Work out the finished part from the listing and answer in its coordinate system (mm). A direction names the side the tool comes from. Coordinates: 2 decimals unless noted, no trailing zeros. Loops run counter-clockwise (first coordinate to the right, second up) from the corner with the lowest first, then second, coordinate; pieces in that order, holes last.
```python
from build123d import *

# Parameters (mm, degrees)
SKETCH1_R           = 3
SKETCH1_R_2         = 8
SKETCH1_R_3         = 1.8
BOSS_EXTRUDE1_DEPTH = 6.2


with BuildPart() as part:
    # Sketch1 → Boss-Extrude1 (new body)
    with BuildSketch(Plane.XY):
        with BuildLine():
            Line((41.889296616, 14.900574245), (50.746753734, 13.965723579))
            ThreePointArc((50.746753734, 13.965723579), (58.138171033, 17.219277376), (59.076989694, 25.240329771))
            ThreePointArc((59.076989694, 25.240329771), (47.870351378, 40.981444556), (31.114327774, 50.604703359))
            ThreePointArc((31.114327774, 50.604703359), (-11.412690469, 54.769217303), (-51.987221097, 41.367802402))
            ThreePointArc((-51.987221097, 41.367802402), (-62.079231834, 16.80974691), (-41, 0.666241851))
            Line((-41, 0.666241851), (-35, 0.666241851))
            ThreePointArc((-35, 0.666241851), (-26.181808949, -1.950576316), (-20.218406631, -8.953865794))
            ThreePointArc((-20.218406631, -8.953865794), (3.76322615, -21.789763842), (22.050412422, -1.653780932))
            ThreePointArc((22.050412422, -1.653780932), (28.467658292, 10.820459281), (41.889296616, 14.900574245))
        make_face()
        with Locations(Location((-41, 22.5, 0), (0, 0, 180))):
            Circle(SKETCH1_R, mode=Mode.SUBTRACT)
        with Locations(Location((6, 41.25, 0), (0, 0, 180))):
            Circle(SKETCH1_R, mode=Mode.SUBTRACT)
        with Locations(Location((51.6, 22.050001086, 0), (0, 0, 180))):
            Circle(SKETCH1_R, mode=Mode.SUBTRACT)
        with Locations(Location((0, 0, 0), (0, 0, 180))):
            Circle(SKETCH1_R_2, mode=Mode.SUBTRACT)
        with Locations(Location((25.2, 42.25, 0), (0, 0, 180))):
            Circle(SKETCH1_R_3, mode=Mode.SUBTRACT)
        with Locations(Location((-32.4, 15.5, 0), (0, 0, 180))):
            Circle(SKETCH1_R_3, mode=Mode.SUBTRACT)
        with Locations(Location((42, 20.450001086, 0), (0, 0, 180))):
            Circle(SKETCH1_R_3, mode=Mode.SUBTRACT)
        with Locations(Location((-41, 33.5, 0), (0, 0, 180))):
            Circle(SKETCH1_R_3, mode=Mode.SUBTRACT)
    extrude(amount=BOSS_EXTRUDE1_DEPTH)


solid = part.part
```
1. A cutting plane is placed at B-B, the plane y = 3. Give the vertices of the cut face in (x, z).
2. Straight lines are drawn through the part: probe 1 along Y at (x, z) = (-41, 1.75); probe 2 along Y at (x, z) = (6, 3); probe 3 along X at (y, z) = (24, 2.75). For each, find the intervals that lie inside material, in ascending order.
3. A cutting plane is placed at D-D, the plane y = 27.5. Give the vertices of the cut face in (x, z), then the cut area to 3 significant figures.
4. A cutting plane is placed at A-A, the plane z = 5.25. Count the separate pieces of the cut face and the enclosed holes in it, then the cut area to 3 significant figures.
5. For faces 4 (the flat face through (-2, 26, 0)), 5 (the flat face through (-38, 0.666, 3)), determine the directions among +Z, -Z, +X, -X, +Y, -Y from which every point of the face is accessible in a straight line to the end or side of a thin tool.
6. A cutting plane is placed at C-C, the plane x = -3. Give the vertices of the cut face in (y, z), then the cut area to 3 significant figures.
7. Determine the mould class of faces 1 (the cylindrical face through (40.283, 19.909, 3.057)), 2 (the flat face through (46.26, 14.44, 3.06)), 3 (the flat face through (-2, 26, 6.2)) for opening direction Y: released by +Y, released by -Y, zero draft, split by the parting line, or undercut.
8. Each of these flat-tipped pins is pushed along its axis until it touches: P1, Ø4, axis at x = 42, y = 20.45, coming from the +Z side; P2, Ø3, axis at x = -37, z = 4, coming from the -Y side; P3, Ø5, axis at x = 51.6, y = 22.05, coming from the +Z side; P4, Ø3, axis at y = 32, z = 4.5, coming from the -X side. Where does it stop, or does it pass through?
Answers below:
1. outline: (-50.82, 0) - (-7.42, 0) - (-7.42, 6.2) - (-50.82, 6.2) - close; (7.42, 0) - (23.03, 0) - (23.03, 6.2) - (7.42, 6.2) - close
2. probe 1: y = 0.67 to 19.5, 25.5 to 31.7, 35.3 to 46.92
2. probe 2: y = -21.28 to -5.29, 5.29 to 38.25, 44.25 to 55.23
2. probe 3: x = -62.78 to -43.6, -38.4 to 49.32, 53.88 to 59.49
3. outline: (-62.25, 0) - (58.04, 0) - (58.04, 6.2) - (-62.25, 6.2) - close
3. area: 746 mm2
4. separate pieces: 1
4. enclosed holes: 8
4. area: 5,730 mm2
5. face 4: -Z, +X, -X, +Y, -Y
5. face 5: +Z, -Z, -X, -Y
6. outline: (-21.91, 0) - (-7.42, 0) - (-7.42, 6.2) - (-21.91, 6.2) - close; (7.42, 0) - (55.36, 0) - (55.36, 6.2) - (7.42, 6.2) - close
6. area: 387 mm2
7. face 1: undercut
7. face 2: released by -Y
7. face 3: zero draft
8. P1: stops at z = 6.2
8. P2: stops at y = 0.67
8. P3: passes through
8. P4: stops at x = -61.32
